Check sheet for the modelled part. Datum: model origin and axes. Units: mm. Face numbers are marked on the shaded views. A direction names the side the tool comes from. Round coordinates to 2 decimals unless told otherwise and drop trailing zeros. Order: outer loops, then holes, each group sorted by start corner. A loop starts at its lowest first (then second) coordinate and runs counter-clockwise, first axis right, second up. Notation, with made-up numbers: (-8, 51) -> (46, 51) arc R16 ccw to (46, 65) -> close; hole circle Ø1 at (22.25, 1). An arc over 180 degrees is marked (long way). Answer in a Markdown table with one row per item.
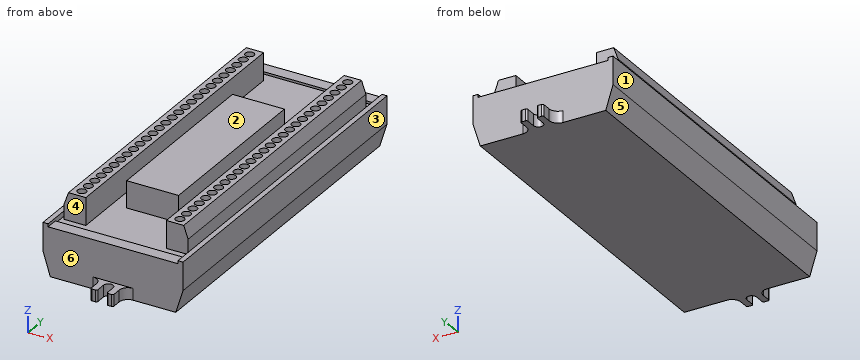
from build123d import *

# Parameters (mm, degrees)
SKETCH1_W           = 48
SKETCH1_H           = 17.6
BOSS_EXTRUDE1_DEPTH = 118.5
SKETCH2_W           = 44.5
SKETCH2_H           = 1
CUT_EXTRUDE1_DEPTH  = 122.225781086
SKETCH3_W           = 44.5
SKETCH3_H           = 110.1
CUT_EXTRUDE2_DEPTH  = 0.8
SKETCH4_W           = 7.75
SKETCH4_H           = 6.5
BOSS_EXTRUDE2_DEPTH = 4
FILLET1_R           = 3
CUT_EXTRUDE3_DEPTH  = 129.494202204
FILLET2_R           = 0.5
SKETCH6_W           = 7.45
SKETCH6_H           = 103.3
BOSS_EXTRUDE3_DEPTH = 9.4
CUT_EXTRUDE4_DEPTH  = 121.945111518
SKETCH8_R           = 1.5
CUT_EXTRUDE5_DEPTH  = 2
SKETCH9_W           = 17.8
SKETCH9_H           = 61.5
BOSS_EXTRUDE4_DEPTH = 9.18


with BuildPart() as part:
    # Sketch1 → Boss-Extrude1 (new body)
    with BuildSketch(Plane(origin=(0, 0, 0), x_dir=(1, 0, 0), z_dir=(0, 1, 0))):
        Rectangle(SKETCH1_W, SKETCH1_H)
    extrude(amount=BOSS_EXTRUDE1_DEPTH)

    # Sketch2 → Cut-Extrude1 (cut, through all)
    with BuildSketch(Plane.XZ):
        with Locations((0, 8.3)):
            Rectangle(SKETCH2_W, SKETCH2_H)
        Polygon((-24, -0.8), (-21.5, -8.8), (-24, -8.8), align=None)
        Polygon((24, -8.8), (21.5, -8.8), (24, -0.8), align=None)
    extrude(amount=-CUT_EXTRUDE1_DEPTH, mode=Mode.SUBTRACT)

    # Sketch3 → Cut-Extrude2 (cut)
    with BuildSketch(Plane.XY.offset(7.8)):
        with Locations((0, 59.25)):
            Rectangle(SKETCH3_W, SKETCH3_H)
    extrude(amount=-CUT_EXTRUDE2_DEPTH, mode=Mode.SUBTRACT)

    # Sketch4 → Boss-Extrude2 (add)
    with BuildSketch(Plane(origin=(0, 0, -8.8), x_dir=(-1, 0, 0), z_dir=(0, 0, -1))):
        with Locations((0, 121.75)):
            Rectangle(SKETCH4_W, SKETCH4_H)
        with Locations((0, -3.25)):
            Rectangle(SKETCH4_W, SKETCH4_H)
    extrude(amount=-BOSS_EXTRUDE2_DEPTH)

    # Fillet1
    fillet1_edges = [part.edges().sort_by_distance(p)[0] for p in [
        (-3.875, 118.5, -6.8),
        (3.875, 118.5, -6.8),
        (3.875, 0, -6.8),
        (-3.875, 0, -6.8),
    ]]
    fillet(fillet1_edges, radius=FILLET1_R)

    # Sketch5 → Cut-Extrude3 (cut, through all)
    with BuildSketch(Plane(origin=(0, 0, -8.8), x_dir=(-1, 0, 0), z_dir=(0, 0, -1))):
        with BuildLine():
            Line((1.65, 129.806526387), (1.65, 121.25))
            ThreePointArc((1.65, 121.25), (0, 119.6), (-1.65, 121.25))
            Line((-1.65, 121.25), (-1.65, 129.806526387))
            ThreePointArc((-1.65, 129.806526387), (0, 131.456526387), (1.65, 129.806526387))
        make_face()
        with BuildLine():
            Line((1.65, -2.75), (1.65, -10.353047519))
            ThreePointArc((1.65, -10.353047519), (0, -12.003047519), (-1.65, -10.353047519))
            Line((-1.65, -10.353047519), (-1.65, -2.75))
            ThreePointArc((-1.65, -2.75), (0, -1.1), (1.65, -2.75))
        make_face()
    extrude(amount=-CUT_EXTRUDE3_DEPTH, mode=Mode.SUBTRACT)

    # Fillet2
    fillet2_edges = [part.edges().sort_by_distance(p)[0] for p in [
        (-1.65, 125, -6.8),
        (1.65, 125, -6.8),
        (-1.65, -6.5, -6.8),
        (1.65, -6.5, -6.8),
        (-3.875, 125, -6.8),
        (3.875, 125, -6.8),
        (3.875, -6.5, -6.8),
        (-3.875, -6.5, -6.8),
    ]]
    fillet(fillet2_edges, radius=FILLET2_R)

    # Sketch6 → Boss-Extrude3 (add)
    with BuildSketch(Plane.XY.offset(7)):
        with Locations((-17.525, 59.25)):
            Rectangle(SKETCH6_W, SKETCH6_H)
        with Locations((17.525, 59.25)):
            Rectangle(SKETCH6_W, SKETCH6_H)
    extrude(amount=BOSS_EXTRUDE3_DEPTH)

    # Sketch7 → Cut-Extrude4 (cut, through all)
    with BuildSketch(Plane.XZ.offset(-7.6)):
        Polygon((-19.75, 16.4), (-21.25, 12.15), (-21.25, 16.4), align=None)
        Polygon((21.25, 16.4), (19.75, 16.4), (21.25, 12.15), align=None)
    extrude(amount=-CUT_EXTRUDE4_DEPTH, mode=Mode.SUBTRACT)

    # Sketch8 → Cut-Extrude5 (cut)
    with BuildSketch(Plane.XY.offset(16.4)):
        with Locations((-16.8, 107.9)):
            Circle(SKETCH8_R)
        with Locations((-16.8, 104.15)):
            Circle(SKETCH8_R)
        with Locations((-16.8, 100.4)):
            Circle(SKETCH8_R)
        with Locations((-16.8, 96.65)):
            Circle(SKETCH8_R)
        with Locations((-16.8, 92.9)):
            Circle(SKETCH8_R)
        with Locations((-16.8, 89.15)):
            Circle(SKETCH8_R)
        with Locations((-16.8, 85.4)):
            Circle(SKETCH8_R)
        with Locations((-16.8, 81.65)):
            Circle(SKETCH8_R)
        with Locations((-16.8, 77.9)):
            Circle(SKETCH8_R)
        with Locations((-16.8, 74.15)):
            Circle(SKETCH8_R)
        with Locations((-16.8, 70.4)):
            Circle(SKETCH8_R)
        with Locations((-16.8, 66.65)):
            Circle(SKETCH8_R)
        with Locations((-16.8, 62.9)):
            Circle(SKETCH8_R)
        with Locations((-16.8, 59.15)):
            Circle(SKETCH8_R)
        with Locations((-16.8, 55.4)):
            Circle(SKETCH8_R)
        with Locations((-16.8, 51.65)):
            Circle(SKETCH8_R)
        with Locations((-16.8, 47.9)):
            Circle(SKETCH8_R)
        with Locations((-16.8, 44.15)):
            Circle(SKETCH8_R)
        with Locations((-16.8, 40.4)):
            Circle(SKETCH8_R)
        with Locations((-16.8, 36.65)):
            Circle(SKETCH8_R)
        with Locations((-16.8, 32.9)):
            Circle(SKETCH8_R)
        with Locations((-16.8, 29.15)):
            Circle(SKETCH8_R)
        with Locations((-16.8, 25.4)):
            Circle(SKETCH8_R)
        with Locations((-16.8, 21.65)):
            Circle(SKETCH8_R)
        with Locations((-16.8, 17.9)):
            Circle(SKETCH8_R)
        with Locations((-16.8, 14.15)):
            Circle(SKETCH8_R)
        with Locations((-16.8, 10.4)):
            Circle(SKETCH8_R)
        with Locations(Location((16.8, 10.4, 0), (0, 0, 180))):
            Circle(SKETCH8_R)
        with Locations(Location((16.8, 14.15, 0), (0, 0, 180))):
            Circle(SKETCH8_R)
        with Locations(Location((16.8, 17.9, 0), (0, 0, 180))):
            Circle(SKETCH8_R)
        with Locations(Location((16.8, 21.65, 0), (0, 0, 180))):
            Circle(SKETCH8_R)
        with Locations(Location((16.8, 25.4, 0), (0, 0, 180))):
            Circle(SKETCH8_R)
        with Locations(Location((16.8, 29.15, 0), (0, 0, 180))):
            Circle(SKETCH8_R)
        with Locations(Location((16.8, 32.9, 0), (0, 0, 180))):
            Circle(SKETCH8_R)
        with Locations(Location((16.8, 36.65, 0), (0, 0, 180))):
            Circle(SKETCH8_R)
        with Locations(Location((16.8, 40.4, 0), (0, 0, 180))):
            Circle(SKETCH8_R)
        with Locations(Location((16.8, 44.15, 0), (0, 0, 180))):
            Circle(SKETCH8_R)
        with Locations(Location((16.8, 47.9, 0), (0, 0, 180))):
            Circle(SKETCH8_R)
        with Locations(Location((16.8, 51.65, 0), (0, 0, 180))):
            Circle(SKETCH8_R)
        with Locations(Location((16.8, 55.4, 0), (0, 0, 180))):
            Circle(SKETCH8_R)
        with Locations(Location((16.8, 59.15, 0), (0, 0, 180))):
            Circle(SKETCH8_R)
        with Locations(Location((16.8, 62.9, 0), (0, 0, 180))):
            Circle(SKETCH8_R)
        with Locations(Location((16.8, 66.65, 0), (0, 0, 180))):
            Circle(SKETCH8_R)
        with Locations(Location((16.8, 70.4, 0), (0, 0, 180))):
            Circle(SKETCH8_R)
        with Locations(Location((16.8, 74.15, 0), (0, 0, 180))):
            Circle(SKETCH8_R)
        with Locations(Location((16.8, 77.9, 0), (0, 0, 180))):
            Circle(SKETCH8_R)
        with Locations(Location((16.8, 81.65, 0), (0, 0, 180))):
            Circle(SKETCH8_R)
        with Locations(Location((16.8, 85.4, 0), (0, 0, 180))):
            Circle(SKETCH8_R)
        with Locations(Location((16.8, 89.15, 0), (0, 0, 180))):
            Circle(SKETCH8_R)
        with Locations(Location((16.8, 92.9, 0), (0, 0, 180))):
            Circle(SKETCH8_R)
        with Locations(Location((16.8, 96.65, 0), (0, 0, 180))):
            Circle(SKETCH8_R)
        with Locations(Location((16.8, 100.4, 0), (0, 0, 180))):
            Circle(SKETCH8_R)
        with Locations(Location((16.8, 104.15, 0), (0, 0, 180))):
            Circle(SKETCH8_R)
        with Locations(Location((16.8, 107.9, 0), (0, 0, 180))):
            Circle(SKETCH8_R)
    extrude(amount=-CUT_EXTRUDE5_DEPTH, mode=Mode.SUBTRACT)

    # Sketch9 → Boss-Extrude4 (add)
    with BuildSketch(Plane.XY.offset(7)):
        with Locations((0.001215362, 53.75)):
            Rectangle(SKETCH9_W, SKETCH9_H)
    extrude(amount=BOSS_EXTRUDE4_DEPTH)


solid = part.part
Item 1: Cross-section at C-C (y = 107.9). Record the boundary of the cut face in (x, z).
Result sheet:
| item | result |
|---|---|
| outline | (-24, -0.8) -> (-21.5, -8.8) -> (21.5, -8.8) -> (24, -0.8) -> (24, 8.8) -> (22.25, 8.8) -> (22.25, 7) -> (21.25, 7) -> (21.25, 12.15) -> (19.75, 16.4) -> (18.3, 16.4) -> (18.3, 14.4) -> (15.3, 14.4) -> (15.3, 16.4) -> (13.8, 16.4) -> (13.8, 7) -> (-13.8, 7) -> (-13.8, 16.4) -> (-15.3, 16.4) -> (-15.3, 14.4) -> (-18.3, 14.4) -> (-18.3, 16.4) -> (-19.75, 16.4) -> (-21.25, 12.15) -> (-21.25, 7) -> (-22.25, 7) -> (-22.25, 8.8) -> (-24, 8.8) -> close |
Item 2: Scan lines: line 1 (X direction, y = 77.9, z = 15.7); line 2 (X direction, y = 77.9, z = 14.8); line 3 (Y direction, x = -21, z = 12.25). Record each from-to range of solid material in increasing order. Write a range as [from, to].
Result sheet:
| item | result |
|---|---|
| line 1 | x = [-20, -18.3], [-15.3, -13.8], [-8.9, 8.9], [13.8, 15.3], [18.3, 20] |
| line 2 | x = [-20.31, -18.3], [-15.3, -13.8], [-8.9, 8.9], [13.8, 15.3], [18.3, 20.31] |
| line 3 | y = [7.6, 110.9] |
Item 3: Set-up check for the marked faces 1 and 2: record each of +Z, -Z, +X, -X, +Y, -Y from which the full face is reachable in a straight line by a thin tool's end or side.
Result sheet:
| item | result |
|---|---|
| face 1 | +Z, -Z, -X, +Y, -Y |
| face 2 | +Z, +Y, -Y |
Item 4: Depth check by flat-ended pin: P1, Ø0.5, axis at x = 23.5, y = 88.5, coming from the +Z side; P2, Ø2, axis at x = 3, y = -2.5, coming from the +Z side; P3, Ø3, axis at x = -18.5, z = 8, coming from the -Y side. Enter the tip coordinate at first touch or a pass-through.
Result sheet:
| item | result |
|---|---|
| P1 | stops at z = 8.8 |
| P2 | stops at z = -4.8 |
| P3 | stops at y = 0 |
Item 5: Mould release check, pull along X, two halves, no side actions. Record for the marked faces 3, 4, 5 and 6: pulls with the +X half, pulls with the -X half, needs draft (parallel to the pull), parting line crosses it, or undercut.
Result sheet:
| item | result |
|---|---|
| face 3 | pulls with the +X half |
| face 4 | undercut |
| face 5 | pulls with the -X half |
| face 6 | needs draft |
Item 6: Cross-section at B-B (x = 12). Record the boundary of the cut face in (y, z).
Result sheet:
| item | result |
|---|---|
| outline | (0, -8.8) -> (118.5, -8.8) -> (118.5, 7.8) -> (114.3, 7.8) -> (114.3, 7) -> (4.2, 7) -> (4.2, 7.8) -> (0, 7.8) -> close |
Item 7: Cross-section at D-D (z = 2). Record the boundary of the cut face in (x, y).
Result sheet:
| item | result |
|---|---|
| outline | (-24, 0) -> (24, 0) -> (24, 118.5) -> (-24, 118.5) -> close |
